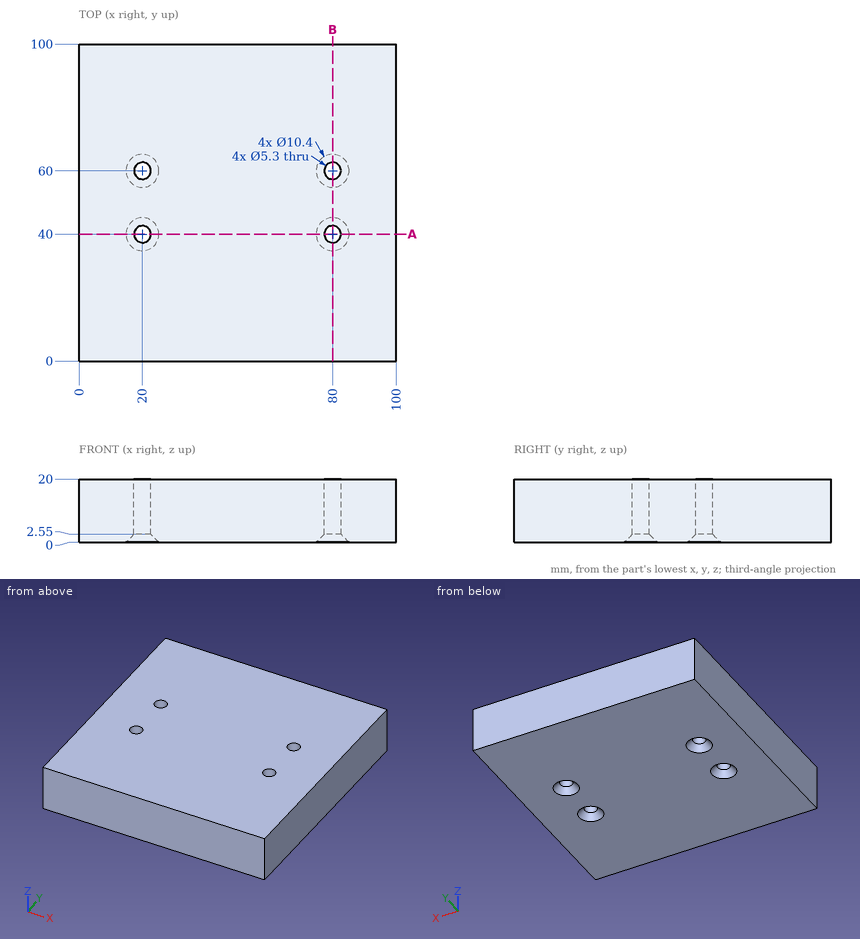
Here's the drawing with two shaded views (mm, measured from the low corner). I have some questions. Coordinates: 2 decimals unless noted, no trailing zeros. Write each loop counter-clockwise with the first axis right and the second up, starting at its lowest first coordinate (ties: lowest second). Pieces come first, ordered by that corner, then holes. Notation, with made-up numbers: M 73,81.25 L 97,81.25 A38 ccw 97,119.25 Z; hole C -30,-4 d4. An arc over 180 degrees is marked long. Answer as CSV lines item,"result". Start each with the question number.
1) I want a section at B-B, the plane x = 80. Please give me the cut outline in (y, z), and give its area (4 significant figures).
2) For P1, Ø1, axis at y = 86, z = 16, coming from the -X side; P2, Ø6, axis at x = 20, y = 60, coming from the -Z side, each with a flat end and sliding along its axis, tell me the tip position at first contact or that it passes through.
3) I want a section at A-A, the plane y = 40. Please give me the cut outline in (x, z).
4) Please list where these lines run through material, in increasing order: line 1 (X direction, y = 40, z = 6.25); line 2 (Y direction, x = 80, z = 15). Write a range as from..to.
Data:
1,outline,"M 0,0 L 34.8,0 L 37.35,2.55 L 37.35,20 L 0,20 Z; M 42.65,2.55 L 45.2,0 L 54.8,0 L 57.35,2.55 L 57.35,20 L 42.65,20 Z; M 62.65,2.55 L 65.2,0 L 100,0 L 100,20 L 62.65,20 Z"
1,area,"1,775 mm^2"
2,P1,"stops at x = 0"
2,P2,"stops at z = 2.2"
3,outline,"M 0,0 L 14.8,0 L 17.35,2.55 L 17.35,20 L 0,20 Z; M 22.65,2.55 L 25.2,0 L 74.8,0 L 77.35,2.55 L 77.35,20 L 22.65,20 Z; M 82.65,2.55 L 85.2,0 L 100,0 L 100,20 L 82.65,20 Z"
4,line 1,"x = 0..17.35, 22.65..77.35, 82.65..100"
4,line 2,"y = 0..37.35, 42.65..57.35, 62.65..100"
